Autodesk Inventor part; units mm, degrees
ref_plane "YZ Plane" through (0, 0, 0) normal (1, 0, 0) x (0, 1, 0)
ref_plane "XZ Plane" through (0, 0, 0) normal (0, 1, 0) x (-1, 0, 0)
ref_plane "XY Plane" through (0, 0, 0) normal (0, 0, 1) x (1, 0, 0)
sketch "Sketch2" plane through (0, 0, 0) normal (0, 1, 0) x (-1, 0, 0)
  point P0 (0, 0)
sketch "Sketch3" plane through (0, 0, 0) normal (0, 1, 0) x (-1, 0, 0)
  line L0 (0, 0) -> (76, 0)
  line L1 (76, 0) -> (76, -76)
  line L2 (76, -76) -> (0, -76)
  line L3 (0, -76) -> (0, 0)
  dimension "d1" = 76
  dimension "d2" = 76
extrude "Extrusion1" add sketch "Sketch3" along normal blind 30
sketch "Sketch4" plane through (0, 30, 0) normal (0, 1, 0) x (1, 0, 0)
  line L0 (-76, 0) -> (0, 0)
  line L1 (0, 0) -> (0, 76)
  line L2 (-23, 23) -> (-53, 23)
  line L3 (-53, 23) -> (-53, 53)
  line L4 (-53, 53) -> (-23, 53)
  line L5 (-23, 53) -> (-23, 23)
  point P0 (-38, 38)
  dimension "d5" = 30
  dimension "d6" = 30
extrude "Extrusion2" add sketch "Sketch4" along normal blind 15
sketch "Sketch5" plane through (-23, 30, -23) normal (1, 0, 0) x (0, 0, -1)
  line L0 (0, 0) -> (0, 15)
  line L1 (30, 0) -> (30, 15)
  line L2 (0, 5.6) -> (30, 5.6)
  line L3 (30, 5.6) -> (30, 9.4)
  line L4 (30, 9.4) -> (0, 9.4)
  line L5 (0, 9.4) -> (0, 5.6)
  point P0 (-23, -30)
  point P1 (15, 7.5)
  dimension "d9" = 3.8
sketch "Sketch6" plane through (-23, 30, -53) normal (0, 0, -1) x (-1, 0, 0)
  line L0 (0, 0) -> (0, 15)
  line L1 (30, 0) -> (30, 15)
  line L2 (0, 5.6) -> (30, 5.6)
  line L3 (30, 5.6) -> (30, 9.4)
  line L4 (30, 9.4) -> (0, 9.4)
  line L5 (0, 9.4) -> (0, 5.6)
  point P0 (-23, -30)
  point P1 (15, 7.5)
  dimension "d10" = 3.8
sketch "Sketch7" plane through (-53, 30, -53) normal (-1, 0, 0) x (0, 0, 1)
  line L0 (0, 0) -> (0, 15)
  line L1 (30, 0) -> (30, 15)
  line L2 (0, 5.6) -> (30, 5.6)
  line L3 (30, 5.6) -> (30, 9.4)
  line L4 (30, 9.4) -> (0, 9.4)
  line L5 (0, 9.4) -> (0, 5.6)
  point P0 (53, -30)
  point P1 (15, 7.5)
  dimension "d11" = 3.8
sketch "Sketch8" plane through (-53, 30, -23) normal (0, 0, 1) x (1, 0, 0)
  line L0 (0, 0) -> (0, 15)
  line L1 (30, 0) -> (30, 15)
  line L2 (0, 5.6) -> (30, 5.6)
  line L3 (30, 5.6) -> (30, 9.4)
  line L4 (30, 9.4) -> (0, 9.4)
  line L5 (0, 9.4) -> (0, 5.6)
  point P0 (53, -30)
  point P1 (15, 7.5)
  dimension "d12" = 3.8
extrude "Extrusion3" cut sketch "Sketch8" against normal blind 2
extrude "Extrusion4" cut sketch "Sketch7" against normal blind 2
extrude "Extrusion5" cut sketch "Sketch6" against normal blind 2
extrude "Extrusion6" cut sketch "Sketch5" against normal blind 2
sketch "Sketch9" plane through (0, 45, 0) normal (0, 1, 0) x (1, 0, 0)
  line L0 (-23, 53) -> (-53, 53)
  line L1 (-53, 23) -> (-23, 23)
  circle A0 centre (-38, 38) radius 12.5
  point P0 (0, 0)
  dimension "d21" = 25
extrude "Extrusion7" cut sketch "Sketch9" against normal blind 25
properties part number "Hydraulic cylinder part 1"
Geometry: final body of the model. Coordinates: model frame, mm. A direction names the side the tool comes from. Round coordinates to 2 decimals unless told otherwise and drop trailing zeros. Loops run counter-clockwise (first coordinate to the right, second up) from the corner with the lowest first, then second, coordinate; pieces in that order, holes last.
Q1. Pull-direction query (X, two-part tool) for faces 1 (the cylindrical face through (-47.92, 32.675, -30.394)), 2 (the flat face through (-38, 33, -23)), 3 (the flat face through (-76, 15, -37)), 4 (the flat face through (-38, 20, -38)); classes: released by +X, released by -X, zero draft, split by the parting line, or undercut.
Q2. Section D-D on y = 32. Return loops of the section in (x, z), plus the area to 3 significant figures.
Q3. Section C-C on z = -38. Return loops of the section in (x, y).
Q4. Section A-A on y = 26.5. Return loops of the section in (x, z).
Q5. Section B-B on x = -38. Return loops of the section in (y, z).
Q6. Pin query (flat end, axial travel): P1, Ø6, axis at y = 35.5, z = -33.5, coming from the -X side; P2, Ø1.7, axis at x = -36, y = 33.5, coming from the -Z side; P3, Ø12.5, axis at x = -40, z = -32.5, coming from the +Y side. Return the tip coordinate at first contact, or that it passes through.
Q7. Access query for faces 5 (the flat face through (-23, 33, -38)), 6 (the flat face through (-38, 38, -51)), 7 (the flat face through (-38, 39.4, -52)). Directions: +Z, -Z, +X, -X, +Y, -Y. A direction counts if a zero-diameter tool reaches every point of the face in a straight line with its end or side. Return the directions, or none.
Q8. Material intervals for L1, parallel to X at y = 26.5, z = -38; L2, parallel to X at y = 34, z = -38; L3, parallel to Y at x = -51.5, z = -37, sorted ascending.
Evaluation:
1. face 1: undercut
1. face 2: zero draft
1. face 3: released by -X
1. face 4: undercut
2. outline: (-53, -53) - (-23, -53) - (-23, -23) - (-53, -23) - close; hole circle Ø25 at (-38, -38)
2. area: 409 mm2
3. outline: (-76, 0) - (0, 0) - (0, 30) - (-23, 30) - (-23, 35.6) - (-25, 35.6) - (-25, 39.4) - (-23, 39.4) - (-23, 45) - (-25.5, 45) - (-25.5, 20) - (-50.5, 20) - (-50.5, 45) - (-53, 45) - (-53, 39.4) - (-51, 39.4) - (-51, 35.6) - (-53, 35.6) - (-53, 30) - (-76, 30) - close
4. outline: (-76, -76) - (0, -76) - (0, 0) - (-76, 0) - close; hole circle Ø25 at (-38, -38)
5. outline: (0, -76) - (30, -76) - (30, -53) - (35.6, -53) - (35.6, -51) - (39.4, -51) - (39.4, -53) - (45, -53) - (45, -50.5) - (20, -50.5) - (20, -25.5) - (45, -25.5) - (45, -23) - (39.4, -23) - (39.4, -25) - (35.6, -25) - (35.6, -23) - (30, -23) - (30, 0) - (0, 0) - close
6. P1: stops at x = -53
6. P2: stops at z = -53
6. P3: stops at y = 20
7. face 5: +Z, -Z, +X, +Y
7. face 6: -Z, +X, -X
7. face 7: none
8. L1: x = -76 to -50.5, -25.5 to 0
8. L2: x = -53 to -50.5, -25.5 to -23
8. L3: y = 0 to 35.6, 39.4 to 45
